from build123d import *

# Parameters (mm, degrees)
F1_DEPTH = 25
F4_DEPTH = 16.8
F6_DEPTH = 1.2
F8_DEPTH = 1.2


with BuildPart() as f1:
    # F0 (on Top) → F1 (new body)
    with BuildSketch(Plane.XY):
        with BuildLine():
            ThreePointArc((-76.5, 0), (0, 76.5), (76.5, 0))
            Line((76.5, 0), (78.5, 0))
            ThreePointArc((78.5, 0), (0, 78.5), (-78.5, 0))
            Line((-78.5, 0), (-76.5, 0))
        make_face()
    extrude(amount=F1_DEPTH)

    # F3 (on offset) → F4 (join)
    with BuildSketch(Plane.XY.offset(4.1)):
        with BuildLine():
            Line((73, 0), (76.5, 0))
            ThreePointArc((76.5, 0), (0, 76.5), (-76.5, 0))
            Line((-76.5, 0), (-73, 0))
            ThreePointArc((-73, 0), (0, 73), (73, 0))
        make_face()
    extrude(amount=F4_DEPTH)

    # F5 (on face) → F6 (join)
    with BuildSketch(Plane.XY.offset(20.9)):
        with BuildLine():
            Line((73, 0), (74.2, 0))
            ThreePointArc((74.2, 0), (0, 74.2), (-74.2, 0))
            Line((-74.2, 0), (-73, 0))
            ThreePointArc((-73, 0), (0, 73), (73, 0))
        make_face()
    extrude(amount=F6_DEPTH)

    # F7 (on face) → F8 (join)
    with BuildSketch(Plane(origin=(0, 0, 4.1), x_dir=(1, 0, 0), z_dir=(0, 0, -1))):
        with BuildLine():
            ThreePointArc((-74.2, 0), (0, -74.2), (74.2, 0))
            Line((74.2, 0), (73, 0))
            ThreePointArc((73, 0), (0, -73), (-73, 0))
            Line((-73, 0), (-74.2, 0))
        make_face()
    extrude(amount=F8_DEPTH)


solid = f1.part
Work out the finished part from the listing and answer in its coordinate system (mm). A direction names the side the tool comes from. Give positions to 0.01 mm unless a question says otherwise; leave off trailing zeros. Order: outer loops, then holes, each group sorted by start corner. A loop starts at its lowest first (then second) coordinate and runs counter-clockwise, first axis right, second up. Notation, with made-up numbers: (43, -28.5) -> (76, -28.5) arc R23 ccw to (76, -19.5) -> close; hole circle Ø9 at (22, 27). An arc over 180 degrees is marked (long way). One line per item, written item: value.
Item 1: Find section A-A, the plane y = 68.5. Give the vertices of the cut face in (x, z), plus the area to 3 significant figures.
Answer sheet:
outline: (-38.34, 0) -> (-34.06, 0) -> (-34.06, 4.1) -> (-28.52, 4.1) -> (-28.52, 2.9) -> (-25.23, 2.9) -> (-25.23, 22.1) -> (-28.52, 22.1) -> (-28.52, 20.9) -> (-34.06, 20.9) -> (-34.06, 25) -> (-38.34, 25) -> close; (25.23, 2.9) -> (28.52, 2.9) -> (28.52, 4.1) -> (34.06, 4.1) -> (34.06, 0) -> (38.34, 0) -> (38.34, 25) -> (34.06, 25) -> (34.06, 20.9) -> (28.52, 20.9) -> (28.52, 22.1) -> (25.23, 22.1) -> close
area: 526 mm²
Item 2: Find section D-D, the plane z = 8. Give the vertices of the cut face in (x, y), plus the area to 3 significant figures.
Answer sheet:
outline: (-78.5, 0) -> (-73, 0) arc R73 cw to (73, 0) -> (78.5, 0) arc R78.5 ccw to start
area: 1,310 mm²
Item 3: Find section C-C, the plane y = 41. Give the vertices of the cut face in (x, z), plus the area to 3 significant figures.
Answer sheet:
outline: (-66.94, 0) -> (-64.59, 0) -> (-64.59, 4.1) -> (-61.84, 4.1) -> (-61.84, 2.9) -> (-60.4, 2.9) -> (-60.4, 22.1) -> (-61.84, 22.1) -> (-61.84, 20.9) -> (-64.59, 20.9) -> (-64.59, 25) -> (-66.94, 25) -> close; (60.4, 2.9) -> (61.84, 2.9) -> (61.84, 4.1) -> (64.59, 4.1) -> (64.59, 0) -> (66.94, 0) -> (66.94, 25) -> (64.59, 25) -> (64.59, 20.9) -> (61.84, 20.9) -> (61.84, 22.1) -> (60.4, 22.1) -> close
area: 265 mm²
Item 4: Determine the mould class of faces 1 (the flat face through (-6, 73, 22.1)), 2 (the cylindrical face through (1.632, 74.182, 21.492)), 3 (the cylindrical face through (1.73, 78.48, 12.32)), 4 (the flat face through (76, 0, 13)) for opening direction Y: released by +Y, released by -Y, zero draft, split by the parting line, or undercut.
Answer sheet:
face 1: zero draft
face 2: undercut
face 3: released by +Y
face 4: released by -Y
Item 5: Find section B-B, the plane x = 0. Give the vertices of the cut face in (y, z), plus the area to 3 significant figures.
Answer sheet:
outline: (73, 2.9) -> (74.2, 2.9) -> (74.2, 4.1) -> (76.5, 4.1) -> (76.5, 0) -> (78.5, 0) -> (78.5, 25) -> (76.5, 25) -> (76.5, 20.9) -> (74.2, 20.9) -> (74.2, 22.1) -> (73, 22.1) -> close
area: 112 mm²
Item 6: Flat-ended cylindrical pins translate along their axes: P1, Ø8, axis at x = 39, z = 6.5, coming from the -Y side; P2, Ø12, axis at y = 36, z = 14, coming from the -X side; P3, Ø1, axis at x = -53.5, z = 17, coming from the -Y side. Find the tip coordinate at first contact, or state that the pin passes through.
Answer sheet:
P1: y = 58.99
P2: x = -72.54
P3: y = 49.12
Item 7: A tool of negligible diameter and unlimited length cuts with its end or side. For faces 5 (the cylindrical face through (-1.68, 76.48, 2.02)), 6 (the flat face through (-76, 0, 13)), 7 (the flat face through (0, 75, 20.9)), 8 (the flat face through (-11, 73, 2.9)), from which of +Z, -Z, +X, -X, +Y, -Y can it reach the whole face along a straight path? Write none if from no direction.
Answer sheet:
face 5: -Z
face 6: +Z, -Z, +X, -X, -Y
face 7: +Z
face 8: -Z, -Y
Item 8: Straight lines are drawn through the part: probe 1 along Z at (x, y) = (2.5, 74); probe 2 along X at (y, z) = (22, 7); probe 3 along X at (y, z) = (63, 16). For each, find the intervals that lie inside material, in ascending order.
Answer sheet:
probe 1: 2.9 to 22.1
probe 2: -75.35 to -69.61, 69.61 to 75.35
probe 3: -46.83 to -36.88, 36.88 to 46.83
